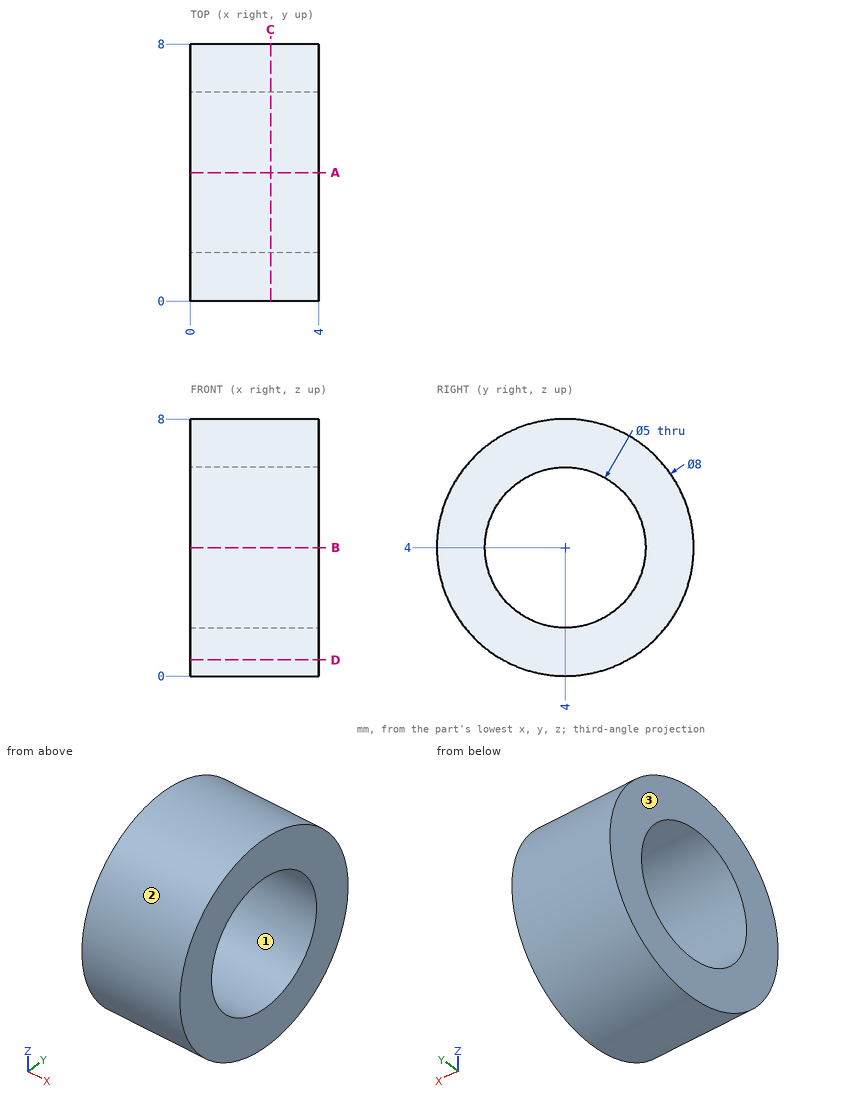
Design review of the part shown in the three views and the two pictorial views. Dimensions are in mm from the part's minimum x, y and z. Give positions to 0.01 mm unless a question says otherwise; leave off trailing zeros. Write each loop counter-clockwise with the first axis right and the second up, starting at its lowest first coordinate (ties: lowest second). Pieces come first, ordered by that corner, then holes. Notation, with made-up numbers: M 0.25,-13.5 L 46.25,-13.5 A6 cw 46.25,-3.5 Z; hole C 23.5,36.25 d3. An arc over 180 degrees is marked long. Return JSON: item names as keys, results as strings. Group by question number.
Item 1: Clearance check with a flat-ended pin moving along its axis: pin 1 Ø2 at (x, z) = (2, 2) entering from +Y. State where the tip first meets the part, or that it passes through.
Item 2: Take a section at C-C (x = 2.5). Give the boundary of the cut face in (y, z).
Item 3: Take a section at D-D (z = 0.5). Give the boundary of the cut face in (x, y).
Item 4: Take a section at A-A (y = 4). Give the boundary of the cut face in (x, z), plus the area to 3 significant figures.
Item 5: Wall thickness on line 1 along Y through (x, z) = (2.6, 4); line 2 along Y through (x, z) = (1.8, 3.25); line 3 along Z through (x, y) = (2.35, 3): over which ranges is each line inside the solid? List them lowest first.
Item 6: The part is to be moulded in two halves that separate along Y. For the marked faces 1, 2 and 3, say which applies: pulls with the +Y half, pulls with the -Y half, needs draft (parallel to the pull), parting line crosses it, or undercut.
Return value:
{
 "1": {"pin 1": "stops at y = 7.87"},
 "2": {"outline": "C 4,4 d8; hole C 4,4 d5"},
 "3": {"outline": "M 0,2.06 L 4,2.06 L 4,5.94 L 0,5.94 Z"},
 "4": {"outline": "M 0,0 L 4,0 L 4,1.5 L 0,1.5 Z; M 0,6.5 L 4,6.5 L 4,8 L 0,8 Z", "area": "12.0 mm2"},
 "5": {"line 1": "y = 0 to 1.5, 6.5 to 8", "line 2": "y = 0.07 to 1.62, 6.38 to 7.93", "line 3": "z = 0.13 to 1.71, 6.29 to 7.87"},
 "6": {"face 1": "undercut", "face 2": "parting line crosses it", "face 3": "needs draft"}
}
